```python
from build123d import *

# Parameters (mm, degrees)
F1_DEPTH  = 104.5
F3_DEPTH  = 127.001
F4_W      = 127
F4_H      = 62
F5_DEPTH  = 27
F7_DEPTH  = 93.5104
F8_W      = 237.597823
F8_H      = 212.603942
F9_DEPTH  = 64.76446
F11_DEPTH = 127.001
F12_DEPTH = 25.4
F13_W     = 127
F13_H     = 18.2746
F14_DEPTH = 28.575
F16_DEPTH = 127.001


with BuildPart() as f1:
    # F0 (on Front) → F1 (new body)
    with BuildSketch(Plane.XZ):
        with BuildLine():
            ThreePointArc((0, 62.5094), (-35.443943, 54.198998), (-63.5, 31))
            Line((-63.5, 31), (0, 31))
            Line((0, 31), (0, 62.5094))
        make_face()
        Polygon((0, 31), (-63.5, 31), (-63.5, -31), (0, -31), (0, 0), align=None)
        with BuildLine():
            Line((0, 62.5094), (0, 31))
            Line((0, 31), (63.5, 31))
            ThreePointArc((63.5, 31), (35.443943, 54.198998), (0, 62.5094))
        make_face()
        Polygon((63.5, 31), (0, 31), (0, 0), (0, -31), (63.5, -31), align=None)
        with BuildLine():
            Line((0, -31), (-63.5, -31))
            ThreePointArc((-63.5, -31), (-35.441854, -54.192308), (0, -62.5))
            Line((0, -62.5), (0, -31))
        make_face()
        with BuildLine():
            Line((63.5, -31), (0, -31))
            Line((0, -31), (0, -62.5))
            ThreePointArc((0, -62.5), (35.441854, -54.192308), (63.5, -31))
        make_face()
    extrude(amount=F1_DEPTH)

    # F2 (on face) → F3 (cut, through all)
    with BuildSketch(Plane.YZ.offset(63.5)):
        Polygon((-104.5, 72.844587), (-104.5, 31), (-62.5, 64.333223), align=None)
        Polygon((-62.5, -65.093011), (-104.5, -31), (-104.5, -67.313612), align=None)
    extrude(amount=-F3_DEPTH, mode=Mode.SUBTRACT)

    # F4 (on face) → F5 (join)
    with BuildSketch(Plane.XZ.offset(104.5)):
        Rectangle(F4_W, F4_H)
    extrude(amount=F5_DEPTH)

    # F6 (on face) → F7 (cut, through all)
    with BuildSketch(Plane(origin=(0, 0, -31), x_dir=(1, 0, 0), z_dir=(0, 0, -1))):
        with BuildLine():
            ThreePointArc((-63.5, 104.5), (-34.500906, 124.469723), (0, 131.5))
            Line((0, 131.5), (-63.5, 131.5))
            Line((-63.5, 131.5), (-63.5, 104.5))
        make_face()
        with BuildLine():
            ThreePointArc((0, 131.5), (34.500906, 124.469723), (63.5, 104.5))
            Line((63.5, 104.5), (63.5, 131.5))
            Line((63.5, 131.5), (0, 131.5))
        make_face()
    extrude(amount=-F7_DEPTH, mode=Mode.SUBTRACT)

    # F8 (on face) → F9 (cut)
    with BuildSketch(Plane(origin=(0, 0, 0), x_dir=(-1, 0, 0), z_dir=(0, 1, 0))):
        with Locations((30.433759, -29.178329)):
            Rectangle(F8_W, F8_H)
    extrude(amount=-F9_DEPTH, mode=Mode.SUBTRACT)

    # F10 (on face) → F11 (cut, through all)
    with BuildSketch(Plane.YZ.offset(63.5)):
        Polygon((-64.76446, -12.7254), (-64.76446, 0), (-64.76446, 76.2), (-148.139939, 76.2), (-148.139939, -12.7254), align=None)
    extrude(amount=-F11_DEPTH, mode=Mode.SUBTRACT)

    # F9_face (on face) → F12 (join)
    with BuildSketch(Plane(origin=(0, -64.76446, -33.868347), x_dir=(-1, 0, 0), z_dir=(0, 1, 0))):
        with BuildLine():
            ThreePointArc((-63.5, 2.868347), (0, -28.631653), (63.5, 2.868347))
            Line((63.5, 2.868347), (63.5, 21.142947))
            Line((63.5, 21.142947), (-63.5, 21.142947))
            Line((-63.5, 21.142947), (-63.5, 2.868347))
        make_face()
    extrude(amount=F12_DEPTH)

    # F13 (on face) → F14 (join)
    with BuildSketch(Plane(origin=(0, -39.36446, 0), x_dir=(-1, 0, 0), z_dir=(0, 1, 0))):
        with BuildLine():
            ThreePointArc((-63.5, -31), (0, -62.5), (63.5, -31))
            Line((63.5, -31), (-63.5, -31))
        make_face()
        with Locations((0, -21.8627)):
            Rectangle(F13_W, F13_H)
    extrude(amount=F14_DEPTH)

    # F15 (on face) → F16 (cut, through all)
    with BuildSketch(Plane(origin=(-63.5, 0, 0), x_dir=(0, -1, 0), z_dir=(-1, 0, 0))):
        Polygon((104.02593, -67.289479), (104.5, -31), (76.034166, -31), (42.225931, -64.199477), align=None)
    extrude(amount=-F16_DEPTH, mode=Mode.SUBTRACT)


solid = f1.part
```
The model under review builds one solid part; all positions refer to its coordinate system, in mm. A direction names the side the tool comes from. Round coordinates to 2 decimals unless told otherwise and drop trailing zeros. Order: outer loops, then holes, each group sorted by start corner. A loop starts at its lowest first (then second) coordinate and runs counter-clockwise, first axis right, second up.
Item 1: For pin 1 (3 mm diameter, centred on x = -4.5, z = -23, fed in from -Y); pin 2 (10 mm diameter, centred on x = 34, y = -85, fed in from -Z); pin 3 (10 mm diameter, centred on x = 1.5, z = -31, fed in from -Y); pin 4 (4 mm diameter, centred on x = -39, y = -47, fed in from -Z), all flat-tipped, find the tip position at first contact; note any pin that passes through.
Working result:
pin 1: stops at y = -131.45
pin 2: stops at z = -31
pin 3: stops at y = -131.5
pin 4: stops at z = -53.4
Item 2: Add section B-B, the plane x = -12. State the section outline as (y, z) points, and give its area (3 significant figures).
Working result:
outline: (-130.68, -31) - (-76.03, -31) - (-44.88, -61.59) - (-10.79, -61.59) - (-10.79, -12.73) - (-130.68, -12.73) - close
area: 3,710 mm2
Item 3: To check wall thickness, follow probe 1 along Z at (x, y) = (22.5, -92); probe 2 along Z at (x, y) = (-21, -30); probe 3 along Y at (x, z) = (-31, -41). State the ranges of each line that lie inside material, in increasing order.
Working result:
probe 1: z = -31 to -12.73
probe 2: z = -59.69 to -12.73
probe 3: y = -65.85 to -10.79
Item 4: Add section A-A, the plane z = -29. State the section outline as (x, y) points.
Working result:
outline: (-63.5, -104.5) arc R88.17 ccw to (0, -131.5) arc R88.17 ccw to (63.5, -104.5) - (63.5, -10.79) - (-63.5, -10.79) - close
Item 5: Add section D-D, the plane y = -94. State the section outline as (x, z) points.
Working result:
outline: (-63.5, -31) - (63.5, -31) - (63.5, -12.73) - (-63.5, -12.73) - close
Item 6: Machinability: for faces 1 (the flat face through (-1, -98, -31)), 2 (the flat face through (1, -72, -12.725)), which of the approach directions +Z, -Z, +X, -X, +Y, -Y give a long, thin tool a straight path to every point of the face, cutting with its end or side? Answer none if there is none.
Working result:
face 1: -Z, +X, -X, -Y
face 2: +Z, +X, -X, +Y, -Y
Item 7: Add section C-C, the plane y = -58. State the section outline as (x, z) points.
Working result:
outline: (-63.5, -31) arc R79.75 ccw to (-44.83, -48.71) - (44.83, -48.71) arc R79.75 ccw to (63.5, -31) - (63.5, -12.73) - (-63.5, -12.73) - close
